Can you work these out from the model? Positions are in its coordinate system, mm. A direction names the side the tool comes from. Round coordinates to 2 decimals unless told otherwise and drop trailing zeros. Loops run counter-clockwise (first coordinate to the right, second up) from the corner with the lowest first, then second, coordinate; pieces in that order, holes last.
(1) Thinking about a two-plate mould opening in Z: for faces 3 (the face through (10, 10, 20)), 4 (the face through (20, 14, 10)), 5 (the face through (10, 8, 8)), 6 (the face through (10, 10, 0)), which applies, released by +Z, released by -Z, zero draft, split by the parting line, or undercut?
(2) Will this pin go through, and if not, where does the flat tip stop? pin 1 Ø1.5 at (y, z) = (17.5, 17) entering from -X.
(3) I want a section at A-A on y = 10. Write out the boundary of the cut face in (x, z).
(4) I want a section at D-D on x = 18.75. Write out the boundary of the cut face in (y, z), plus the area to 3 significant figures.
(5) If I drill on line 1 along Y through (x, z) = (4.5, 10); line 2 along Y through (x, z) = (15.25, 10); line 3 along Z through (x, y) = (17.75, 9.75), over which ranges is the centre line in solid material (lowest first)?
(6) Which directions (+Z, -Z, +X, -X, +Y, -Y) give clear straight access to the entire face, cutting with the end or side of a thin tool? Please do faces 1 (the face through (5, 12, 10)), 2 (the face through (15.07, 6.583, 10.759)).
(7) I want a section at B-B on x = 9. Write out the boundary of the cut face in (y, z), plus the area to 3 significant figures.
Autodesk Inventor part; units mm, degrees
ref_plane "YZ Plane" through (0, 0, 0) normal (1, 0, 0) x (0, 1, 0)
ref_plane "XZ Plane" through (0, 0, 0) normal (0, 1, 0) x (-1, 0, 0)
ref_plane "XY Plane" through (0, 0, 0) normal (0, 0, 1) x (1, 0, 0)
sketch "Sketch1" plane through (0, 0, 0) normal (0, 0, 1) x (1, 0, 0)
  line L0 (0, 0) -> (20, 0)
  line L1 (20, 0) -> (20, 20)
  line L2 (20, 20) -> (0, 20)
  line L3 (0, 20) -> (0, 0)
  line L4 (0, 20) -> (10, 20)
  dimension "d0" = 20
  dimension "d1" = 20
extrude "Extrusion1" add sketch "Sketch1" along normal blind 20
sketch "Sketch2" plane through (20, 0, 0) normal (1, 0, 0) x (0, 0, -1)
  circle A0 centre (-10, 10) radius 3.5
  line L0 (0, 20) -> (-20, 20)
  line L1 (-20, 0) -> (-20, 20)
  point P0 (0, 0)
  dimension "d4" = 7
  dimension "d5" = 10
  dimension "d6" = 10
extrude "Extrusion2" cut sketch "Sketch2" against normal blind 10
sketch "Sketch3" plane through (0, 0, 0) normal (-1, 0, 0) x (0, 0, 1)
  circle A0 centre (10, 10) radius 2
  line L0 (0, 0) -> (20, 0)
  line L1 (20, 20) -> (20, 0)
  dimension "d9" = 4
  dimension "d10" = 10
  dimension "d11" = 10
extrude "Extrusion3" cut sketch "Sketch3" against normal blind 10
properties part number "holetest"
Filled sheet:
1. face 3: released by +Z
1. face 4: zero draft
1. face 5: undercut
1. face 6: released by -Z
2. pin 1: stops at x = 0
3. outline: (0, 0) - (20, 0) - (20, 6.5) - (10, 6.5) - (10, 8) - (0, 8) - close; (0, 12) - (10, 12) - (10, 13.5) - (20, 13.5) - (20, 20) - (0, 20) - close
4. outline: (0, 0) - (20, 0) - (20, 20) - (0, 20) - close; hole circle Ø7 at (10, 10)
4. area: 362 mm2
5. line 1: y = 0 to 8, 12 to 20
5. line 2: y = 0 to 6.5, 13.5 to 20
5. line 3: z = 0 to 6.51, 13.49 to 20
6. face 1: +X, -X
6. face 2: +X
7. outline: (0, 0) - (20, 0) - (20, 20) - (0, 20) - close; hole circle Ø4 at (10, 10)
7. area: 387 mm2
